Verification items for the finished model (mm, model axes). A direction names the side the tool comes from. Coordinates: 2 decimals unless noted, no trailing zeros. Write each loop counter-clockwise with the first axis right and the second up, starting at its lowest first coordinate (ties: lowest second). Pieces come first, ordered by that corner, then holes. Notation, with made-up numbers: (18.25, 73.25) -> (38.25, 73.25) arc R27 cw to (38.25, 94.25) -> close; hole circle Ø11 at (42, -39). An arc over 180 degrees is marked (long way). Answer in a Markdown table with one row per item.
```python
from build123d import *

# Parameters (mm, degrees)
SKETCH_1_R         = 5.95
EXTRUDE_1_DEPTH    = 22
SKETCH_2_R         = 5.4
EXTRUDE_2_DEPTH    = 1
SKETCH_3_R         = 5.95
EXTRUDE_3_DEPTH    = 1
HOLE_WIZARD_M3_2_D = 2.5


with BuildPart() as part:
    # 草图1 → 凸台-拉伸1 (new body)
    with BuildSketch(Plane(origin=(0, 0, 0), x_dir=(1, 0, 0), z_dir=(0, 1, 0))):
        with Locations(Location((5.9, 0, 0), (0, 0, 270))):
            Circle(SKETCH_1_R)
    extrude_1 = extrude(amount=EXTRUDE_1_DEPTH)

    # 草图2 → 凸台-拉伸2 (add)
    with BuildSketch(Plane(origin=(0, 22, 0), x_dir=(1, 0, 0), z_dir=(0, 1, 0))):
        with Locations(Location((5.9, 0, 0), (0, 0, 270))):
            Circle(SKETCH_2_R)
    extrude_2 = extrude(amount=EXTRUDE_2_DEPTH)

    # 草图3 → 凸台-拉伸3 (add)
    with BuildSketch(Plane(origin=(0, 23, 0), x_dir=(1, 0, 0), z_dir=(0, 1, 0))):
        with Locations(Location((5.9, 0, 0), (0, 0, 270))):
            Circle(SKETCH_3_R)
    extrude_3 = extrude(amount=EXTRUDE_3_DEPTH)

    # 镜向10: 凸台-拉伸1, 凸台-拉伸2, 凸台-拉伸3 across plane
    add(extrude_1.mirror(Plane.ZX))
    add(extrude_2.mirror(Plane.ZX))
    add(extrude_3.mirror(Plane.ZX))

    # M3 螺纹孔2 (through all)
    with Locations(Plane(origin=(-0.05, -8, 0), x_dir=(0, 0, -1), z_dir=(-1, 0, 0))):
        with Locations((0, 0), (0, -16)):
            Hole(HOLE_WIZARD_M3_2_D / 2)


solid = part.part
```
1. Sectioned sample at D-D, the plane y = 8. Record the cut outline in (x, z), and give its area (3 significant figures).
Findings below:
| item | result |
|---|---|
| outline | (0.08, -1.25) arc R5.95 ccw to (11.72, -1.25) -> close; (0.08, 1.25) -> (11.72, 1.25) arc R5.95 ccw to start |
| area | 81.7 mm² |
2. Sectioned sample at B-B, the plane z = 0. Record the cut outline in (x, y), and give its area (4 significant figures).
Findings below:
| item | result |
|---|---|
| outline | (-0.05, -24) -> (11.85, -24) -> (11.85, -23) -> (11.3, -23) -> (11.3, -22) -> (11.85, -22) -> (11.85, -9.25) -> (-0.05, -9.25) -> (-0.05, -22) -> (0.5, -22) -> (0.5, -23) -> (-0.05, -23) -> close; (-0.05, -6.75) -> (11.85, -6.75) -> (11.85, 6.75) -> (-0.05, 6.75) -> close; (-0.05, 9.25) -> (11.85, 9.25) -> (11.85, 22) -> (11.3, 22) -> (11.3, 23) -> (11.85, 23) -> (11.85, 24) -> (-0.05, 24) -> (-0.05, 23) -> (0.5, 23) -> (0.5, 22) -> (-0.05, 22) -> close |
| area | 509.5 mm² |
3. Go/stop test with flat-tipped pins: pin 1 (5 mm diameter, centred on x = 3, y = 11.5, fed in from +Z); pin 2 (6 mm diameter, centred on y = 7, z = -1.5, fed in from +X); pin 3 (2 mm diameter, centred on y = -5, z = 2, fed in from -X); pin 4 (2 mm diameter, centred on y = 8, z = 0, fed in from -X). Record where each tip stops, or that it passes through.
Findings below:
| item | result |
|---|---|
| pin 1 | stops at z = 5.94 |
| pin 2 | stops at x = 11.85 |
| pin 3 | stops at x = 0.03 |
| pin 4 | passes through |
4. Material ranges on probe 1 along Y at (x, z) = (6.5, 0); probe 2 along Y at (x, z) = (10, -1); probe 3 along Z at (x, y) = (10, -9), recorded low to high. Write a range as from..to.
Findings below:
| item | result |
|---|---|
| probe 1 | y = -24..-9.25, -6.75..6.75, 9.25..24 |
| probe 2 | y = -24..-8.75, -7.25..7.25, 8.75..24 |
| probe 3 | z = -4.31..-0.75, 0.75..4.31 |
5. Access from +Z, -Z, +X, -X, +Y, -Y to the whole of each face (thin tool, end or side, straight path). Record for faces 5 (the face through (1, -23, 3)), 6 (the face through (11.8, 23.49, -0.77)).
Findings below:
| item | result |
|---|---|
| face 5 | none |
| face 6 | +Y, -Y |
6. Sectioned sample at A-A, the plane x = 5.9. Record the cut outline in (y, z).
Findings below:
| item | result |
|---|---|
| outline | (-24, -5.95) -> (-23, -5.95) -> (-23, -5.4) -> (-22, -5.4) -> (-22, -5.95) -> (22, -5.95) -> (22, -5.4) -> (23, -5.4) -> (23, -5.95) -> (24, -5.95) -> (24, 5.95) -> (23, 5.95) -> (23, 5.4) -> (22, 5.4) -> (22, 5.95) -> (-22, 5.95) -> (-22, 5.4) -> (-23, 5.4) -> (-23, 5.95) -> (-24, 5.95) -> close; hole circle Ø2.5 at (-8, 0); hole circle Ø2.5 at (8, 0) |
7. Release check for a two-part mould opening along Y. For faces 1 (the face through (11.8, -23.49, -0.77)), 2 (the face through (6, 24, 0)), 3 (the face through (6, -24, 0)), 4 (the face through (5.98, -6.78, -0.27)) record: released by +Y, released by -Y, zero draft, split by the parting line, or undercut.
Findings below:
| item | result |
|---|---|
| face 1 | zero draft |
| face 2 | released by +Y |
| face 3 | released by -Y |
| face 4 | undercut |
8. Sectioned sample at C-C, the plane z = -3.25. Record the cut outline in (x, y), and give its area (3 significant figures).
Findings below:
| item | result |
|---|---|
| outline | (0.92, -24) -> (10.88, -24) -> (10.88, -23) -> (10.21, -23) -> (10.21, -22) -> (10.88, -22) -> (10.88, 22) -> (10.21, 22) -> (10.21, 23) -> (10.88, 23) -> (10.88, 24) -> (0.92, 24) -> (0.92, 23) -> (1.59, 23) -> (1.59, 22) -> (0.92, 22) -> (0.92, -22) -> (1.59, -22) -> (1.59, -23) -> (0.92, -23) -> close |
| area | 476 mm² |
